from build123d import *

# Parameters (mm, degrees)
BOSS_EXTRUDE1_DEPTH = 432
CUT_EXTRUDE1_DEPTH  = 23
SKETCH3_W           = 15
SKETCH3_H           = 25
CUT_EXTRUDE2_DEPTH  = 3


with BuildPart() as part:
    # Sketch1 → Boss-Extrude1 (new body)
    with BuildSketch(Plane.XY):
        Polygon((0, 0), (20, 0), (20, 2), (2, 2), (2, 20), (0, 20), align=None)
    extrude(amount=BOSS_EXTRUDE1_DEPTH)

    # Sketch2 → Cut-Extrude1 (cut, symmetric)
    with BuildSketch(Plane(origin=(0, 2, 0), x_dir=(1, 0, 0), z_dir=(0, 1, 0))):
        Polygon((0, -432), (20, -432), (0, -412), align=None)
        Polygon((20, 0), (0, -20), (0, 0), align=None)
    extrude(amount=CUT_EXTRUDE1_DEPTH, both=True, mode=Mode.SUBTRACT)

    # Sketch3 → Cut-Extrude2 (cut, through all)
    with BuildSketch(Plane(origin=(0, 2, 0), x_dir=(1, 0, 0), z_dir=(0, 1, 0))):
        with Locations((12.5, -93.5)):
            Rectangle(SKETCH3_W, SKETCH3_H)
        with Locations((12.5, -338.5)):
            Rectangle(SKETCH3_W, SKETCH3_H)
    extrude(amount=-CUT_EXTRUDE2_DEPTH, mode=Mode.SUBTRACT)


solid = part.part
Could you check a few things on this model? Use its own coordinates, in mm. A direction names the side the tool comes from. Give positions to 0.01 mm unless a question says otherwise; leave off trailing zeros. Loops run counter-clockwise (first coordinate to the right, second up) from the corner with the lowest first, then second, coordinate; pieces in that order, holes last. Notation, with made-up numbers: (47, -17) -> (85, -17) arc R25 cw to (85, 16) -> close; hole circle Ø7 at (-30.5, -30). An arc over 180 degrees is marked (long way). Answer as CSV lines item,"result". Start each with the question number.
(1) I need wall thicknesses on probe 1 along X at (y, z) = (9.5, 102); probe 2 along Z at (x, y) = (11, 1.5). Which ranges of each line are inside material? Lowest first, please.
(2) If we section it at C-C on y = 9.5: Write out the boundary of the cut face in (x, z), then the cut area to 3 significant figures.
(3) I'm going to push flat-ended pins straight in: pin 1 Ø0.6 at (x, y) = (12.5, 0.5) entering from +Z; pin 2 Ø5 at (x, z) = (14.5, 160) entering from -Y; pin 3 Ø1.6 at (x, y) = (15.5, 1) entering from +Z; pin 4 Ø1.6 at (y, z) = (1, 93) entering from +X. Where does each tip first touch, or does it pass through?
(4) Which directions (+Z, -Z, +X, -X, +Y, -Y) give clear straight access to the entire face, cutting with the end or side of a thin tool? Please do faces 1 (the flat face through (11, 2, 213)), 2 (the flat face through (0, 10, 213)).
(5) If we section it at A-A on x = 15.5: Write out the boundary of the cut face in (y, z).
(6) If we section it at B-B on z = 94.5: Write out the boundary of the cut face in (x, y).
(7) If we section it at D-D on z = 222.5: Write out the boundary of the cut face in (x, y), then the cut area to 3 significant figures.
Computed:
1,probe 1,"x = 0 to 2"
1,probe 2,"z = 9 to 81, 106 to 326, 351 to 423"
2,outline,"(0, 20) -> (2, 18) -> (2, 414) -> (0, 412) -> close"
2,area,"788 mm2"
3,pin 1,"stops at z = 424.8"
3,pin 2,"stops at y = 0"
3,pin 3,"stops at z = 428.3"
3,pin 4,"stops at x = 5"
4,face 1,"+Z, -Z, +X, +Y"
4,face 2,"+Z, -Z, -X, +Y, -Y"
5,outline,"(0, 4.5) -> (2, 4.5) -> (2, 81) -> (0, 81) -> close; (0, 106) -> (2, 106) -> (2, 326) -> (0, 326) -> close; (0, 351) -> (2, 351) -> (2, 427.5) -> (0, 427.5) -> close"
6,outline,"(0, 0) -> (5, 0) -> (5, 2) -> (2, 2) -> (2, 20) -> (0, 20) -> close"
7,outline,"(0, 0) -> (20, 0) -> (20, 2) -> (2, 2) -> (2, 20) -> (0, 20) -> close"
7,area,"76.0 mm2"
